Input: part model. Units: mm. Frame: model coordinates. Face numbers are marked on the shaded views. Give positions to 0.01 mm unless a question says otherwise; leave off trailing zeros. Loops run counter-clockwise (first coordinate to the right, second up) from the corner with the lowest first, then second, coordinate; pieces in that order, holes last. Notation, with made-up numbers: (44, -24.75) - (98, -24.75) arc R20 ccw to (98, -1.75) - close; hole circle Ø11 at (-17.75, 38). An arc over 180 degrees is marked (long way). Answer as a JSON object with one key per item and string values.
from build123d import *

# Parameters (mm, degrees)
F0_W      = 83
F0_H      = 35
F1_DEPTH  = 3
F6_R      = 2.5
F7_DEPTH  = 15
F3_R      = 2.5
F8_DEPTH  = 15
F4_R      = 2.5
F9_DEPTH  = 15
F10_DEPTH = 15
F5_R      = 2.5
F11_DEPTH = 15


with BuildPart() as f1:
    # F0 (on Front) → F1 (new body)
    with BuildSketch(Plane.XZ):
        Rectangle(F0_W, F0_H)
    extrude(amount=F1_DEPTH)

    # F6 (on face) → F7 (join)
    with BuildSketch(Plane.XZ.offset(3)):
        with Locations((-39.1526, -15.285481)):
            Circle(F6_R)
    extrude(amount=F7_DEPTH)

    # F3 (on face) → F8 (join)
    with BuildSketch(Plane.XZ.offset(3)):
        with Locations((-39.057095, 15.556678)):
            Circle(F3_R)
    extrude(amount=F8_DEPTH)

    # F4 (on face) → F9 (join)
    with BuildSketch(Plane.XZ.offset(3)):
        with Locations((38.984798, 15.55259)):
            Circle(F4_R)
    extrude(amount=F9_DEPTH)

    # F6 (on face) → F10 (join)
    with BuildSketch(Plane.XZ.offset(3)):
        with Locations((-39.1526, -15.285481)):
            Circle(F6_R)
    extrude(amount=F10_DEPTH)

    # F5 (on face) → F11 (join)
    with BuildSketch(Plane.XZ.offset(3)):
        with Locations((38.981859, -15.430422)):
            Circle(F5_R)
    extrude(amount=F11_DEPTH)


solid = f1.part
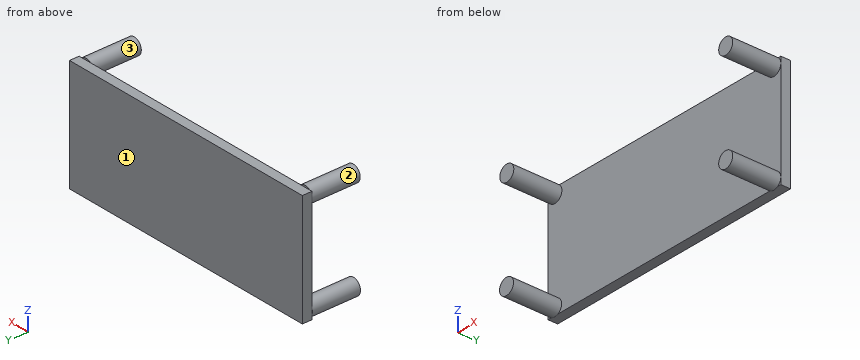
Item 1: Contact query for flat-ended pins moving along their axis: P1, Ø8, axis at x = 22.5, z = -12.5, coming from the -Y side; P2, Ø3.5, axis at x = 17.5, y = -1, coming from the +Z side; P3, Ø3.5, axis at y = -2, z = 7, coming from the -X side; P4, Ø4, axis at y = -6.5, z = -4, coming from the +X side (3 decimals). Output: stop coordinate, or through.
Geometry check:
{"P1": "stops at y = -3", "P2": "stops at z = 17.5", "P3": "stops at x = -41.5", "P4": "passes through"}
Item 2: Cut plane C-C (x = -5.5). Return loops of the section in (y, z).
Geometry check:
{"outline": "(-3, -17.5) - (0, -17.5) - (0, 17.5) - (-3, 17.5) - close"}
Item 3: Material intervals for line 1 (X direction, y = -13.5, z = 15.5); line 2 (Y direction, x = 31, z = 15.5); line 3 (X direction, y = -2, z = -11.5), sorted ascending. Write a range as [from, to].
Geometry check:
{"line 1": "x = [-41.56, -36.56], [36.49, 41.48]", "line 2": "y = [-3, 0]", "line 3": "x = [-41.5, 41.5]"}
Item 4: Cut plane B-B (z = 14). Return loops of the section in (x, y).
Geometry check:
{"outline": "(-41.5, -3) - (-41.01, -3) - (-41.01, -18) - (-37.1, -18) - (-37.1, -3) - (37.03, -3) - (37.03, -18) - (40.94, -18) - (40.94, -3) - (41.5, -3) - (41.5, 0) - (-41.5, 0) - close"}
Item 5: Cut plane A-A (y = -10.25). Return loops of the section in (x, z), then the cut area to 3 significant figures.
Geometry check:
{"outline": "circle Ø5 at (-39.15, -15.29); circle Ø5 at (-39.06, 15.56); circle Ø5 at (38.98, -15.43); circle Ø5 at (38.98, 15.55)", "area": "78.5 mm2"}
Item 6: Cut plane D-D (z = 3). Return loops of the section in (x, y).
Geometry check:
{"outline": "(-41.5, -3) - (41.5, -3) - (41.5, 0) - (-41.5, 0) - close"}
Item 7: Mould query, pull axis Z, two halves, no side actions, for the marked faces 1, 2 and 3. Classes: released by +Z, released by -Z, zero draft, split by the parting line, or undercut.
Geometry check:
{"face 1": "zero draft", "face 2": "undercut", "face 3": "undercut"}
